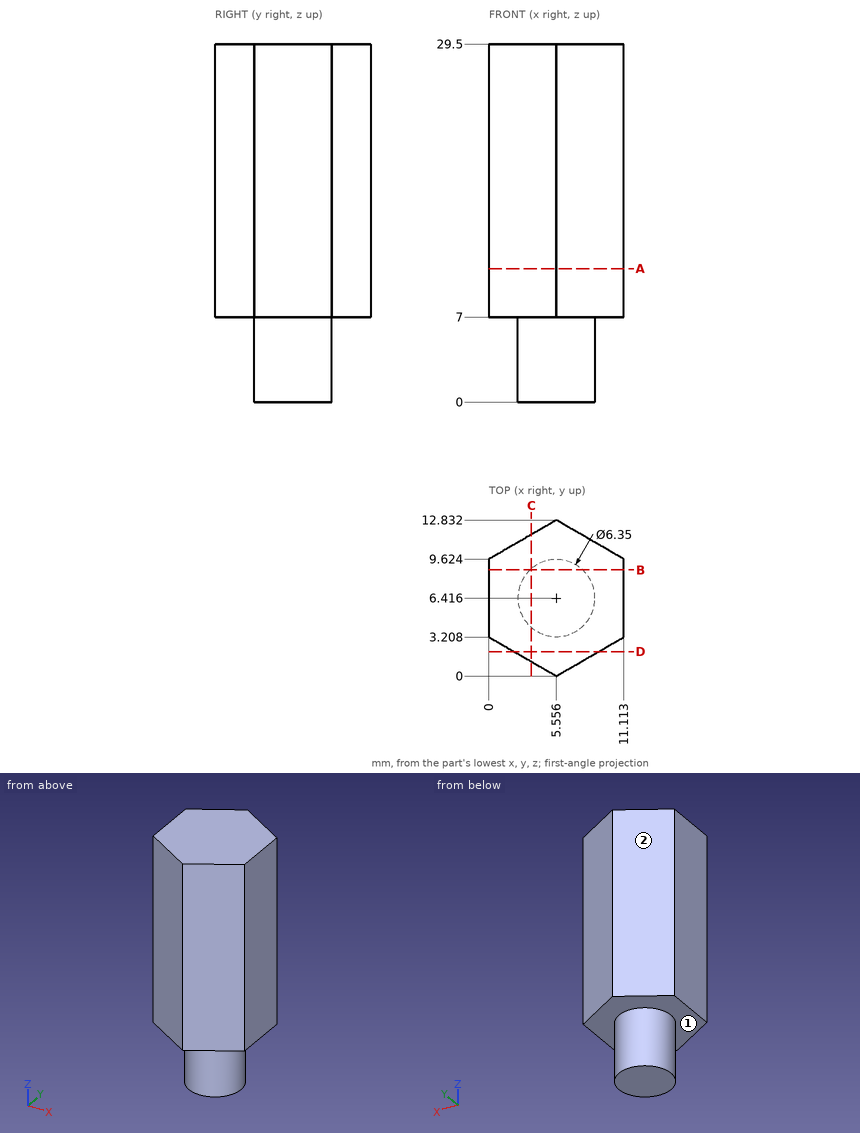
For this review, use the dimensioned drawing (mm, ordinates from the lowest corner) and the shaded views. A direction names the side the tool comes from. Round coordinates to 2 decimals unless told otherwise and drop trailing zeros. Write each loop counter-clockwise with the first axis right and the second up, starting at its lowest first coordinate (ties: lowest second). Pieces come first, ordered by that corner, then holes. Notation, with made-up numbers: (-8, -6.75) - (13, -6.75) arc R17 ccw to (13, 3.25) - close; hole circle Ø11 at (11.25, 51.25). An arc over 180 degrees is marked (long way). One line per item, written item: value. Start each with the question number.
1. Consider section C-C on x = 3.5. Write out the cut boundary in (y, z) (1 decimal).
2. Clearance check with a flat-ended pin moving along its axis: P1, Ø1, axis at x = 5.5, z = 3.5, coming from the +Y side. State where the tip first meets the part, or that it passes through.
3. To check wall thickness, follow L1, parallel to Z at x = 0.75, y = 3.5; L2, parallel to X at y = 11, z = 14.75 (1 decimal); L3, parallel to X at y = 7.5, z = 4.5. State the ranges of each line that lie inside material, in increasing order. Write a range as from..to.
4. Machinability: for the marked faces 1 and 2, which of the approach directions +Z, -Z, +X, -X, +Y, -Y give a long, thin tool a straight path to every point of the face, cutting with its end or side? Answer none if there is none.
5. Consider section A-A on z = 11. Write out the cut boundary in (x, y), and give its area (3 significant figures).
6. Consider section B-B on y = 8.75. Write out the cut boundary in (x, z) (1 decimal), and give its area (3 significant figures).
7. Consider section D-D on y = 2. Write out the cut boundary in (x, z).
Checks:
1. outline: (1.2, 7) - (4, 7) - (4, 0) - (8.8, 0) - (8.8, 7) - (11.6, 7) - (11.6, 29.5) - (1.2, 29.5) - close
2. P1: stops at y = 9.59
3. L1: z = 7..29.5
3. L2: x = 2.4..8.7
3. L3: x = 2.57..8.54
4. face 1: -Z
4. face 2: +Z, -Z, -X, +Y
5. outline: (0, 3.21) - (5.56, 0) - (11.11, 3.21) - (11.11, 9.62) - (5.56, 12.83) - (0, 9.62) - close
5. area: 107 mm^2
6. outline: (0, 7) - (3.4, 7) - (3.4, 0) - (7.7, 0) - (7.7, 7) - (11.1, 7) - (11.1, 29.5) - (0, 29.5) - close
6. area: 280 mm^2
7. outline: (2.09, 7) - (9.02, 7) - (9.02, 29.5) - (2.09, 29.5) - close
